The listing builds one solid part. Answer for the finished solid, in the listing's coordinates (mm). A direction names the side the tool comes from. Give positions to 0.01 mm unless a question says otherwise; leave off trailing zeros. Order: outer loops, then holes, each group sorted by start corner. A loop starts at its lowest first (then second) coordinate and runs counter-clockwise, first axis right, second up.
```python
from build123d import *

# Parameters (mm, degrees)
F1_DEPTH = 15
F2_T     = -2
F3_DEPTH = 2
F5_DEPTH = 2
F6_W     = 10.1464129984
F6_H     = 12.3371165246
F7_DEPTH = 3


with BuildPart() as f1:
    # F0 (on Top) → F1 (new body)
    with BuildSketch(Plane.XY):
        Polygon((7.0000002384, 15), (7.0000002384, 75), (4.5000002384, 75), (-5, 75), (-7.5, 75), (-7.5, 15), (-23.5152803361, 15), (-23.5152803361, -70), (-21, -70), (21, -70), (23.7875375897, -70), (23.7875375897, 15), (21, 15), align=None)
    extrude(amount=-F1_DEPTH)

    # F2
    f2_openings = [f1.faces().sort_by_distance(p)[0] for p in [
        (0.067441, -14.603177, 0),
    ]]
    offset(amount=F2_T, openings=f2_openings, kind=Kind.INTERSECTION)

    # F0 (on Top) → F3 (join)
    with BuildSketch(Plane.XY):
        Polygon((-26, -75), (26, -75), (26, 20), (9.5000002384, 20), (9.5000002384, 75), (7.0000002384, 75), (7.0000002384, 15), (21, 15), (23.7875375897, 15), (23.7875375897, -70), (21, -70), (-21, -70), (-23.5152803361, -70), (-23.5152803361, 15), (-7.5, 15), (-7.5, 75), (-10, 75), (-10, 20), (-26, 20), align=None)
    extrude(amount=-F3_DEPTH)

    # F4 (on face) → F5 (cut)
    with BuildSketch(Plane(origin=(0, 0, -15), x_dir=(1, 0, 0), z_dir=(0, 0, -1))):
        Polygon((23.7875375897, 70), (-23.5152803361, 70), (-23.5152803361, -15), (-7.5, -15), (7.0000002384, -15), (23.7875375897, -15), align=None)
    extrude(amount=-F5_DEPTH, mode=Mode.SUBTRACT)

    # F6 (on face) → F7 (cut)
    with BuildSketch(Plane(origin=(0, 75, 0), x_dir=(-1, 0, 0), z_dir=(0, 1, 0))):
        with Locations((0, -6.1685582623)):
            Rectangle(F6_W, F6_H)
    extrude(amount=-F7_DEPTH, mode=Mode.SUBTRACT)


solid = f1.part
```
1) Find section B-B (y = 17.5). Write down the section's boundary in (x, z).
Geometry says:
outline: (-26, -2) - (-7.5, -2) - (-7.5, -15) - (7, -15) - (7, -2) - (26, -2) - (26, 0) - (5, 0) - (5, -13) - (-5.5, -13) - (-5.5, 0) - (-26, 0) - close
2) Find section C-C (y = -16.5). Write down the section's boundary in (x, z), then the cut area to 3 significant figures.
Geometry says:
outline: (-26, -2) - (-23.52, -2) - (-23.52, -13) - (-21.52, -13) - (-21.52, 0) - (-26, 0) - close; (21.79, -13) - (23.79, -13) - (23.79, -2) - (26, -2) - (26, 0) - (21.79, 0) - close
area: 61.4 mm2
3) Find section D-D (z = -8.75). Write down the section's boundary in (x, y), then the cut area to 3 significant figures.
Geometry says:
outline: (-23.52, -70) - (23.79, -70) - (23.79, 15) - (7, 15) - (7, 75) - (5.07, 75) - (5.07, 72) - (5, 72) - (5, 13) - (21.79, 13) - (21.79, -68) - (-21.52, -68) - (-21.52, 13) - (-5.5, 13) - (-5.5, 73) - (-5.07, 73) - (-5.07, 75) - (-7.5, 75) - (-7.5, 15) - (-23.52, 15) - close
area: 733 mm2
4) A tool of negligible diameter and unlimited length cuts with its end or side. For faces 4 (the flat face through (23.788, -28, -7)), 5 (the flat face through (-7.5, 45, -8)), 6 (the flat face through (-5.5, 43, -6)), 7 (the flat face through (16, 15, -7)), 8 (the flat face through (14, 13, -6)), from which of +Z, -Z, +X, -X, +Y, -Y can it reach the whole face along a straight path? Write none if from no direction.
Geometry says:
face 4: -Z, +X, +Y, -Y
face 5: -Z, -X, +Y
face 6: +Z
face 7: -Z, +X, +Y
face 8: +Z, -Z
5) Given P1, Ø3.5, axis at y = -17.5, z = -9, coming from the +X side; P2, Ø6.5, axis at y = 52, z = -10, coming from the +X side; P3, Ø9, axis at x = 15.5, z = -9.5, coming from the +Y side, each flat-ended and moving along its own axis, determine where each tip first touches the part or whether it passes through.
Geometry says:
P1: stops at x = 23.79
P2: stops at x = 7
P3: stops at y = 15
6) Straight lines are drawn through the part: probe 1 along X at (y, z) = (47, -7); probe 2 along X at (y, z) = (5, -5.75); probe 3 along Y at (x, z) = (-21, -3.25). For each, find the intervals that lie inside material, in ascending order.
Geometry says:
probe 1: x = -7.5 to -5.5, 5 to 7
probe 2: x = -23.52 to -21.52, 21.79 to 23.79
probe 3: y = -70 to -68, 13 to 15
7) For a pull along Y with two mould halves and no side action, classify faces 1 (the flat face through (-21.515, -27, -6)), 2 (the flat face through (0, -70, -7)), 3 (the flat face through (7, 45, -8)) as +Y half, -Y half, draft (parallel to the pull), parting line (faces both ways), or undercut.
Geometry says:
face 1: undercut
face 2: -Y half
face 3: draft
8) Find section A-A (x = 11). Write down the section's boundary in (y, z), then the cut area to 3 significant figures.
Geometry says:
outline: (-75, -2) - (-70, -2) - (-70, -13) - (-68, -13) - (-68, 0) - (-75, 0) - close; (13, -13) - (15, -13) - (15, -2) - (20, -2) - (20, 0) - (13, 0) - close
area: 72.0 mm2
